from build123d import *

# Parameters (mm, degrees)
SKETCH1_W           = 500
SKETCH1_H           = 50
BOSS_EXTRUDE1_DEPTH = 10
SKETCH2_R           = 2.5
CUT_EXTRUDE1_DEPTH  = 10


with BuildPart() as part:
    # Sketch1 → Boss-Extrude1 (new body)
    with BuildSketch(Plane(origin=(0, 0, 0), x_dir=(1, 0, 0), z_dir=(0, 1, 0))):
        with Locations((250, -25)):
            Rectangle(SKETCH1_W, SKETCH1_H)
    extrude(amount=BOSS_EXTRUDE1_DEPTH)

    # Sketch2 → Cut-Extrude1 (cut)
    with BuildSketch(Plane(origin=(0, 10, 0), x_dir=(1, 0, 0), z_dir=(0, 1, 0))):
        with Locations((4.2, -16.1)):
            Circle(SKETCH2_R)
        with Locations((4.2, -33.9)):
            Circle(SKETCH2_R)
        with Locations((495.8, -33.9)):
            Circle(SKETCH2_R)
        with Locations((495.8, -16.1)):
            Circle(SKETCH2_R)
        Polygon((0, -25), (0, -22.5), (8, -22.5), (8, -27.5), (0, -27.5), align=None)
        Polygon((500, -27.5), (500, -25), (500, -22.5), (492, -22.5), (492, -27.5), align=None)
    extrude(amount=-CUT_EXTRUDE1_DEPTH, mode=Mode.SUBTRACT)


solid = part.part
Input: part model. Units: mm. Frame: model coordinates. A direction names the side the tool comes from. Coordinates: 2 decimals unless noted, no trailing zeros. Answer as a JSON object with one key per item and string values. Group by question number.
(1) Set-up query: faces 5 (the face through (4, 5, 22.5)), 6 (the face through (496, 5, 22.5)), 7 (the face through (500, 5, 39)). Return all of +Z, -Z, +X, -X, +Y, -Y with unobstructed straight access to the full face (end or side cutting, diameter ignored); none if empty.
(2) Ray query, line 1 along Z through (x, y) = (495.8, 8); line 2 along X through (y, z) = (4.5, 16.1); line 3 along X through (y, z) = (2.25, 15.5). Return the intervals inside material, ascending. Write a range as [from, to].
(3) Mould query, pull axis Z, two halves, no side actions, for faces 1 (the face through (247, 5, 0)), 2 (the face through (496, 5, 27.5)), 3 (the face through (4, 5, 27.5)), 4 (the face through (247, 0, 25)). Classes: pulls with the +Z half, pulls with the -Z half, needs draft (parallel to the pull), parting line crosses it, or undercut.
Result set:
{
 "1": {"face 5": "-X, +Y, -Y", "face 6": "+X, +Y, -Y", "face 7": "+Z, -Z, +X, +Y, -Y"},
 "2": {"line 1": "z = [0, 13.6], [18.6, 22.5], [27.5, 31.4], [36.4, 50]", "line 2": "x = [0, 1.7], [6.7, 493.3], [498.3, 500]", "line 3": "x = [0, 1.77], [6.63, 493.37], [498.23, 500]"},
 "3": {"face 1": "pulls with the -Z half", "face 2": "undercut", "face 3": "undercut", "face 4": "needs draft"}
}
